Autodesk Inventor part; units mm, degrees
ref_plane "YZ Plane" through (0, 0, 0) normal (1, 0, 0) x (0, 1, 0)
ref_plane "XZ Plane" through (0, 0, 0) normal (0, 1, 0) x (-1, 0, 0)
ref_plane "XY Plane" through (0, 0, 0) normal (0, 0, 1) x (1, 0, 0)
sketch "Sketch1" plane through (0, 0, 0) normal (0, 1, 0) x (-1, 0, 0)
  point P0 (0, 0)
sketch "Sketch2" plane through (0, 0, 0) normal (0, 1, 0) x (-1, 0, 0)
  line L0 (0, 0) -> (57, 0)
  line L1 (57, 0) -> (57, -61)
  line L2 (57, -61) -> (0, -61)
  line L3 (0, -61) -> (0, 0)
  line L4 (67, -71) -> (67, 10)
  line L5 (67, 10) -> (-10, 10)
  line L6 (-10, 10) -> (-10, -71)
  line L7 (-10, -71) -> (67, -71)
  dimension "d0" = 57
  dimension "d1" = 61
  dimension "d2" = 10
extrude "Extrusion1" add sketch "Sketch2" along normal blind 2
sketch "Sketch3" plane through (0, 2, 0) normal (0, 1, 0) x (1, 0, 0)
  line L0 (10, -10) -> (10, 71)
  line L1 (-67, 71) -> (-67, -10)
  line L2 (10, -10) -> (-67, -10)
  line L3 (-67, -10) -> (-67, 71)
  line L4 (-67, 71) -> (10, 71)
  line L5 (10, 71) -> (10, -10)
  line L6 (6, 67) -> (-63, 67)
  line L7 (-63, 67) -> (-63, -6)
  line L8 (-63, -6) -> (6, -6)
  line L9 (6, -6) -> (6, 67)
  point P0 (0, 0)
  dimension "d5" = 4
extrude "Extrusion2" add sketch "Sketch3" along normal blind 2
properties part number "Scannframebottom"
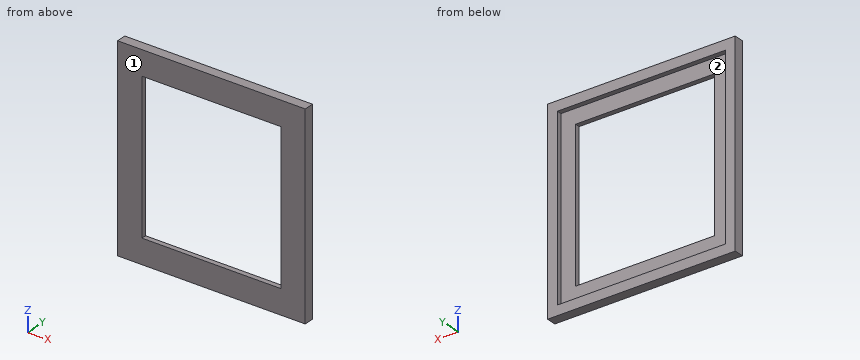
Work out the finished part from the listing and answer in its coordinate system (mm). Face numbers are marked on the shaded views. Coordinates: 2 decimals unless noted, no trailing zeros. Write each loop counter-clockwise with the first axis right and the second up, starting at its lowest first coordinate (ties: lowest second). Pieces come first, ordered by that corner, then holes. Notation, with made-up numbers: M 65,61 L 106,61 A12 ccw 106,82 Z; hole C -37.5,31 d2. An arc over 180 degrees is marked long. Answer as CSV lines item,"result". Start each with the question number.
Item 1: Determine the mould class of the marked faces 1 and 2 for opening direction Z: released by +Z, released by -Z, zero draft, split by the parting line, or undercut.
Item 2: Section B-B on z = -1 is taken. Write down the section's boundary in (x, y).
Item 3: Section D-D on x = 5 is taken. Write down the section's boundary in (y, z).
Item 4: Section C-C on y = 0.7 is taken. Write down the section's boundary in (x, z).
Item 5: Section A-A on x = -8.5 is taken. Write down the section's boundary in (y, z).
Item 6: Consider L1, parallel to X at y = 2.4, z = -14; L2, parallel to Z at x = -26.5, y = 0.75; L3, parallel to X at y = 1.1, z = -15.5. Determine where each line is inside the solid, lowest interval first.
Checks:
1,face 1,"zero draft"
1,face 2,"undercut"
2,outline,"M -67,0 L -57,0 L -57,2 L -63,2 L -63,4 L -67,4 Z; M 0,0 L 10,0 L 10,4 L 6,4 L 6,2 L 0,2 Z"
3,outline,"M 0,-71 L 4,-71 L 4,-67 L 2,-67 L 2,6 L 4,6 L 4,10 L 0,10 Z"
4,outline,"M -67,-71 L 10,-71 L 10,10 L -67,10 Z; hole M -57,-61 L 0,-61 L 0,0 L -57,0 Z"
5,outline,"M 0,-71 L 4,-71 L 4,-67 L 2,-67 L 2,-61 L 0,-61 Z; M 0,0 L 2,0 L 2,6 L 4,6 L 4,10 L 0,10 Z"
6,L1,"x = -67 to -63, 6 to 10"
6,L2,"z = -71 to -61, 0 to 10"
6,L3,"x = -67 to -57, 0 to 10"
